Design review of the part built by this model. Coordinates are the model's own, in mm. Face numbers are marked on the shaded views. A direction names the side the tool comes from. Coordinates: 2 decimals unless noted, no trailing zeros. Write each loop counter-clockwise with the first axis right and the second up, starting at its lowest first coordinate (ties: lowest second). Pieces come first, ordered by that corner, then holes.
Q1. Take a section at B-B (z = 0). Give the boundary of the cut face in (x, y) (3 decimals), and give its area (3 significant figures).
Q2. Take a section at D-D (x = -7). Give the boundary of the cut face in (y, z) (3 decimals).
Q3. Mouldability with a two-part tool opening along Z and no side actions: class the marked faces 3, 4, 5 and 6 as pulls with the +Z half, pulls with the -Z half, needs draft (parallel to the pull), parting line crosses it, or undercut.
Q4. Machinability: for the marked faces 1 and 2, which of the approach directions +Z, -Z, +X, -X, +Y, -Y give a long, thin tool a straight path to every point of the face, cutting with its end or side? Answer none if there is none.
Q5. Insertion check: pin 1 (6 mm diameter, centred on x = 3, z = 6.5, fed in from -Y) (3 decimals); pin 2 (1 mm diameter, centred on x = -2, y = 3, fed in from -Z). Each pin has a flat end and moves straight along its axis. Give the tip position at first contact, or say it passes through.
Q6. Take a section at C-C (y = 3.5). Give the boundary of the cut face in (x, z).
Q7. Take a section at A-A (x = 0). Give the boundary of the cut face in (y, z) (3 decimals), and give its area (3 significant figures).
Q8. For probe 1 along Z at (x, y) = (0.5, 4.25); probe 2 along Y at (x, z) = (-4.75, -6.25) (3 decimals); probe 3 along Z at (x, y) = (7, 0.25), list the stretches that pass through material, from the lowest coordinate up.
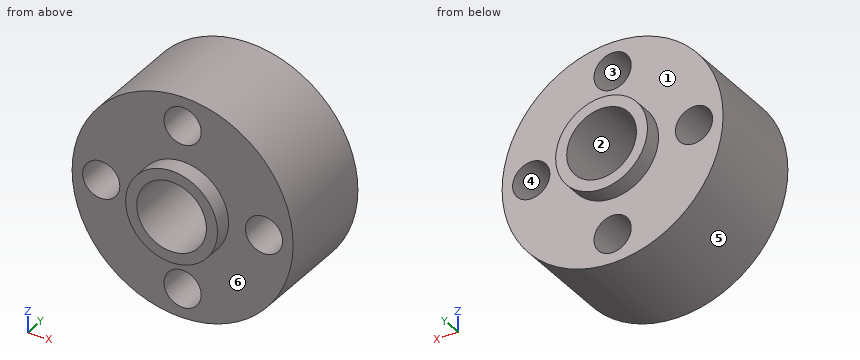
```python
from build123d import *

# Parameters (mm, degrees)
SKETCH_1_W                  = 9.5
SKETCH_1_H                  = 8.8
SKETCH_2_R                  = 3.95
EXTRUDE_1_DEPTH             = 1.5
EXTRUDE_START               = 1.5
SKETCH_3_R                  = 3.95
EXTRUDE_2_DEPTH             = 1.5
HOLE_WIZARD_3_2_3_2_1_D     = 3.2
HOLE_WIZARD_3_2_3_2_1_DEPTH = 10.3
HOLE_WIZARD_6_0_6_1_D       = 6


with BuildPart() as part:
    # 草图1 → 旋转1 (revolve)
    with BuildSketch(Plane(origin=(0, 0, 0), x_dir=(-1, 0, 0), z_dir=(0, 0, -1)), mode=Mode.PRIVATE) as revolve_1_sk:
        with Locations((-4.75, 0.025)):
            Rectangle(SKETCH_1_W, SKETCH_1_H)
    revolve(revolve_1_sk.sketch.rotate(Axis((0, -4.375, 0), (0, 1, 0)), 270), axis=Axis((0, -4.375, 0), (0, 1, 0)))

    # 草图2 → 凸台-拉伸1 (add)
    with BuildSketch(Plane(origin=(0, 4.425, 0), x_dir=(-1, 0, 0), z_dir=(0, 1, 0))):
        with Locations(Location((0, 0, 0), (0, 0, 90))):
            Circle(SKETCH_2_R)
    extrude(amount=EXTRUDE_1_DEPTH)

    # 草图3 → 凸台-拉伸2 (add)
    with BuildSketch(Plane.XZ.offset(4.375).offset(EXTRUDE_START)):
        with Locations(Location((0, 0, 0), (0, 0, 90))):
            Circle(SKETCH_3_R)
    extrude(amount=-EXTRUDE_2_DEPTH)

    # Ø3.2 (3.2) 直径孔1
    with Locations(Plane(origin=(0, -4.375, 0), x_dir=(-1, 0, 0), z_dir=(0, -1, 0))):
        with Locations((0, 7), (-7, 0), (0, -7), (7, 0)):
            Hole(HOLE_WIZARD_3_2_3_2_1_D / 2, depth=HOLE_WIZARD_3_2_3_2_1_DEPTH)

    # Ø6.0 (6) 直径孔1 (through all)
    with Locations(Plane(origin=(0, -5.875, 0), x_dir=(-1, 0, 0), z_dir=(0, -1, 0))):
        with Locations((0, 0)):
            Hole(HOLE_WIZARD_6_0_6_1_D / 2)


solid = part.part
```
Response:
1. outline: (-9.5, -4.375) - (-8.6, -4.375) - (-8.6, 4.425) - (-9.5, 4.425) - close; (-5.4, -4.375) - (-3.95, -4.375) - (-3.95, -5.875) - (-3, -5.875) - (-3, 5.925) - (-3.95, 5.925) - (-3.95, 4.425) - (-5.4, 4.425) - close; (3, -5.875) - (3.95, -5.875) - (3.95, -4.375) - (5.4, -4.375) - (5.4, 4.425) - (3.95, 4.425) - (3.95, 5.925) - (3, 5.925) - close; (8.6, -4.375) - (9.5, -4.375) - (9.5, 4.425) - (8.6, 4.425) - close
1. area: 63.8 mm2
2. outline: (-4.375, -6.423) - (4.425, -6.423) - (4.425, -1.6) - (-4.375, -1.6) - close; (-4.375, 1.6) - (4.425, 1.6) - (4.425, 6.423) - (-4.375, 6.423) - close
3. face 3: undercut
3. face 4: undercut
3. face 5: parting line crosses it
3. face 6: needs draft
4. face 1: +Y
4. face 2: +Y, -Y
5. pin 1: stops at y = -4.375
5. pin 2: stops at z = -9.38
6. outline: circle Ø19 at (0, 0); hole circle Ø3.2 at (-7, 0); hole circle Ø6 at (0, 0); hole circle Ø3.2 at (0, -7); hole circle Ø3.2 at (0, 7); hole circle Ø3.2 at (7, 0)
7. outline: (-5.875, -3.95) - (-4.375, -3.95) - (-4.375, -5.4) - (4.425, -5.4) - (4.425, -3.95) - (5.925, -3.95) - (5.925, -3) - (-5.875, -3) - close; (-5.875, 3) - (5.925, 3) - (5.925, 3.95) - (4.425, 3.95) - (4.425, 5.4) - (-4.375, 5.4) - (-4.375, 3.95) - (-5.875, 3.95) - close; (-4.375, -9.5) - (4.425, -9.5) - (4.425, -8.6) - (-4.375, -8.6) - close; (-4.375, 8.6) - (4.425, 8.6) - (4.425, 9.5) - (-4.375, 9.5) - close
7. area: 63.8 mm2
8. probe 1: z = -9.49 to -8.52, -5.48 to -2.96, 2.96 to 5.48, 8.52 to 9.49
8. probe 2: y = -4.375 to 4.425
8. probe 3: z = -6.42 to -1.6, 1.6 to 6.42
